```python
from build123d import *

# Parameters (mm, degrees)
BOSS_EXTRUDE1_DEPTH                                 = 25.4
CSK_FOR_1_4_FLAT_HEAD_MACHINE_SCREW_100_D           = 6.7564
CSK_FOR_1_4_FLAT_HEAD_MACHINE_SCREW_100_DEPTH       = 16.51
CSK_FOR_1_4_FLAT_HEAD_MACHINE_SCREW_100_CSINK_D     = 12.8778
CSK_FOR_1_4_FLAT_HEAD_MACHINE_SCREW_100_CSINK_ANGLE = 100
CSK_FOR_1_4_FLAT_HEAD_MACHINE_SCREW_100_TIP         = 2.029827343
CSK_FOR_1_4_FLAT_HEAD_MACHINE_SCREW_2_D             = 6.7564
CSK_FOR_1_4_FLAT_HEAD_MACHINE_SCREW_2_DEPTH         = 16.51
CSK_FOR_1_4_FLAT_HEAD_MACHINE_SCREW_2_CSINK_D       = 12.8778
CSK_FOR_1_4_FLAT_HEAD_MACHINE_SCREW_2_CSINK_ANGLE   = 100
CSK_FOR_1_4_FLAT_HEAD_MACHINE_SCREW_2_TIP           = 2.029827343


with BuildPart() as part:
    # Sketch1 → Boss-Extrude1 (new body)
    with BuildSketch(Plane(origin=(0, 0, 0), x_dir=(1, 0, 0), z_dir=(0, 1, 0))):
        Polygon((-1.6, 0), (1.6, 0), (1.6, 25), (13.6, 25), (13.6, -8), (-9.6, -8), (-9.6, 19), (-34.6, 19), (-34.6, 25), (-1.6, 25), align=None)
    extrude(amount=BOSS_EXTRUDE1_DEPTH)

    # Sketch3 → 1/4-20 Tapped Hole1 (revolve, cut)
    with BuildSketch(Plane(origin=(-1.6, 12.7, -12.5), x_dir=(0, 0, -1), z_dir=(0, 1, 0))):
        Polygon((0, 0), (0, 18.043816902), (2.5527, 16.51), (2.5527, 0), align=None)
    revolve(axis=Axis((4.75, 12.7, -12.5), (-1, 0, 0)), mode=Mode.SUBTRACT)

    # CSK for 1_4 Flat Head Machine Screw _100
    with Locations(Plane(origin=(13.6, 0, 0), x_dir=(0, 0, -1), z_dir=(1, 0, 0))):
        with Locations((12.5, 12.7)):
            CounterSinkHole(CSK_FOR_1_4_FLAT_HEAD_MACHINE_SCREW_100_D / 2, CSK_FOR_1_4_FLAT_HEAD_MACHINE_SCREW_100_CSINK_D / 2, depth=CSK_FOR_1_4_FLAT_HEAD_MACHINE_SCREW_100_DEPTH, counter_sink_angle=CSK_FOR_1_4_FLAT_HEAD_MACHINE_SCREW_100_CSINK_ANGLE)
            with Locations((0, 0, -(CSK_FOR_1_4_FLAT_HEAD_MACHINE_SCREW_100_DEPTH + CSK_FOR_1_4_FLAT_HEAD_MACHINE_SCREW_100_TIP / 2))):  # 118° drill point
                Cone(0, CSK_FOR_1_4_FLAT_HEAD_MACHINE_SCREW_100_D / 2, CSK_FOR_1_4_FLAT_HEAD_MACHINE_SCREW_100_TIP, mode=Mode.SUBTRACT)

    # CSK for 1_4 Flat Head Machine Screw  2
    with Locations(Plane.XY.offset(-19)):
        with Locations((-22.1, 12.7)):
            CounterSinkHole(CSK_FOR_1_4_FLAT_HEAD_MACHINE_SCREW_2_D / 2, CSK_FOR_1_4_FLAT_HEAD_MACHINE_SCREW_2_CSINK_D / 2, depth=CSK_FOR_1_4_FLAT_HEAD_MACHINE_SCREW_2_DEPTH, counter_sink_angle=CSK_FOR_1_4_FLAT_HEAD_MACHINE_SCREW_2_CSINK_ANGLE)
            with Locations((0, 0, -(CSK_FOR_1_4_FLAT_HEAD_MACHINE_SCREW_2_DEPTH + CSK_FOR_1_4_FLAT_HEAD_MACHINE_SCREW_2_TIP / 2))):  # 118° drill point
                Cone(0, CSK_FOR_1_4_FLAT_HEAD_MACHINE_SCREW_2_D / 2, CSK_FOR_1_4_FLAT_HEAD_MACHINE_SCREW_2_TIP, mode=Mode.SUBTRACT)


solid = part.part
```
Work out the finished part from the listing and answer in its coordinate system (mm). A direction names the side the tool comes from. Give positions to 0.01 mm unless a question says otherwise; leave off trailing zeros. Order: outer loops, then holes, each group sorted by start corner. A loop starts at its lowest first (then second) coordinate and runs counter-clockwise, first axis right, second up. Notation, with made-up numbers: (20, -30.75) - (27, -30.75) arc R17 cw to (27, -7.75) - close; hole circle Ø10 at (80.25, 2). An arc over 180 degrees is marked (long way). One line per item, written item: value. Start each with the question number.
1. For a pull along Z with two mould halves and no side action, classify faces 4 (the face through (-6.46, 14.965, -13.678)), 5 (the face through (-18, 13, -25)), 6 (the face through (-16, 10, -19)) as released by +Z, released by -Z, zero draft, split by the parting line, or undercut.
2. Section D-D, the plane z = -1 is taken. Write down the section's boundary in (x, y).
3. Section B-B, the plane y = 12.7 is taken. Count the separate pieces of the cut face and the enclosed holes in it, then the cut area to 3 significant figures.
4. Section A-A, the plane x = -22.1 is taken. Write down the section's boundary in (y, z).
5. Consider line 1 (X direction, y = 15.5, z = -3); line 2 (Y direction, x = -8, z = -12.5); line 3 (Z direction, x = -7.25, y = 12.7). Determine where each line is inside the solid, lowest interval first.
6. Section C-C, the plane z = -12.5 is taken. Write down the section's boundary in (x, y).
7. Each of these flat-tipped pins is pushed along its axis until it touches: pin 1 Ø7.5 at (y, z) = (10.5, -5.5) entering from -X; pin 2 Ø10 at (y, z) = (12, -15) entering from +X; pin 3 Ø1 at (x, y) = (0, 19) entering from -Z; pin 4 Ø7.5 at (x, y) = (-23, 11) entering from +Z. Where does it stop, or does it pass through?
8. Which of the six approach directions +Z, -Z, +X, -X, +Y, -Y give full straight-line access (tool end or side, diameter ignored) to faces 1 (the face through (1.6, 15.3, -9.5)), 2 (the face through (6.25, 10.644, -15.181)), 3 (the face through (-9.6, 13, -5))?
Filled sheet:
1. face 4: undercut
1. face 5: released by -Z
1. face 6: released by +Z
2. outline: (-9.6, 0) - (-1.6, 0) - (-1.6, 25.4) - (-9.6, 25.4) - close; (1.6, 0) - (13.6, 0) - (13.6, 25.4) - (1.6, 25.4) - close
3. separate pieces: 4
3. enclosed holes: 0
3. area: 655 mm²
4. outline: (0, -25) - (9.32, -25) - (9.32, -21.57) - (6.26, -19) - (0, -19) - close; (16.08, -25) - (25.4, -25) - (25.4, -19) - (19.14, -19) - (16.08, -21.57) - close
5. line 1: -9.6 to -1.6, 1.6 to 13.6
5. line 2: 0 to 10.15, 15.25 to 25.4
5. line 3: -25 to -15.05, -9.95 to 8
6. outline: (-9.6, 0) - (-1.6, 0) - (-1.6, 9.32) - (-2.91, 9.32) - (-3.41, 10.15) - (-9.6, 10.15) - close; (-9.6, 15.25) - (-3.41, 15.25) - (-2.91, 16.08) - (-1.6, 16.08) - (-1.6, 25.4) - (-9.6, 25.4) - close; (1.6, 0) - (13.6, 0) - (13.6, 6.26) - (11.03, 9.32) - (1.6, 9.32) - close; (1.6, 16.08) - (11.03, 16.08) - (13.6, 19.14) - (13.6, 25.4) - (1.6, 25.4) - close
7. pin 1: x = -9.6
7. pin 2: x = 13.6
7. pin 3: z = 0
7. pin 4: z = -19.64
8. face 1: -Z, +Y, -Y
8. face 2: +X
8. face 3: +Z, -X, +Y, -Y
